Verification items for this drawing (mm, ordinates from the low corner). Give positions to 0.01 mm unless a question says otherwise; leave off trailing zeros. Loops run counter-clockwise (first coordinate to the right, second up) from the corner with the lowest first, then second, coordinate; pieces in that order, holes last. Notation, with made-up numbers: (46, 30.25) -> (50, 30.25) arc R11 cw to (50, 40.25) -> close; hole circle Ø11 at (77, 0.5). An arc over 180 degrees is marked (long way). Write item = value, one per line.
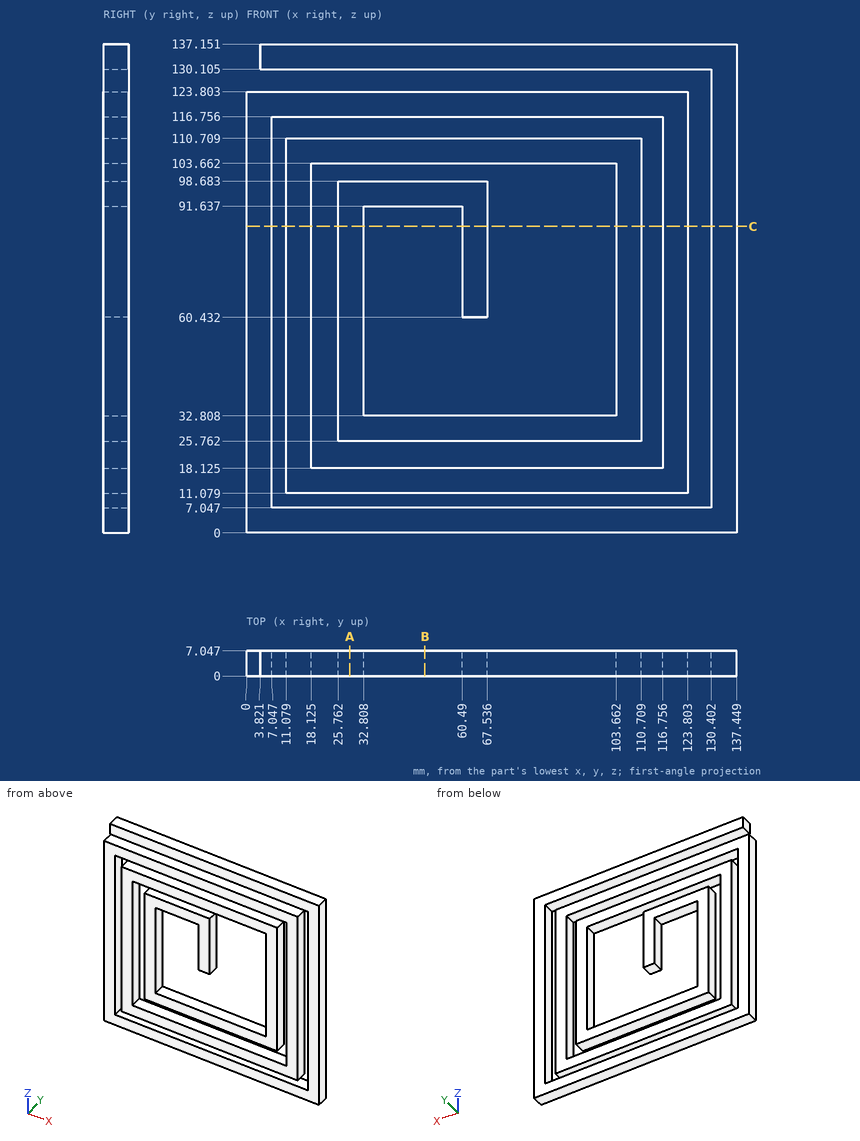
Item 1: Section check B-B, the plane x = 50. Record the cut outline in (y, z) (1 decimal).
Answer:
outline = (0, 0) -> (7, 0) -> (7, 7) -> (0, 7) -> close; (0, 11.1) -> (7, 11.1) -> (7, 18.1) -> (0, 18.1) -> close; (0, 25.8) -> (7, 25.8) -> (7, 32.8) -> (0, 32.8) -> close; (0, 91.6) -> (7, 91.6) -> (7, 98.7) -> (0, 98.7) -> close; (0, 103.7) -> (7, 103.7) -> (7, 110.7) -> (0, 110.7) -> close; (0, 116.8) -> (7, 116.8) -> (7, 123.8) -> (0, 123.8) -> close; (0, 130.1) -> (7, 130.1) -> (7, 137.2) -> (0, 137.2) -> close
Item 2: Section check A-A, the plane x = 29. Record the cut outline in (y, z) (1 decimal), plus the area to 3 significant figures.
Answer:
outline = (0, 0) -> (7, 0) -> (7, 7) -> (0, 7) -> close; (0, 11.1) -> (7, 11.1) -> (7, 18.1) -> (0, 18.1) -> close; (0, 25.8) -> (7, 25.8) -> (7, 98.7) -> (0, 98.7) -> close; (0, 103.7) -> (7, 103.7) -> (7, 110.7) -> (0, 110.7) -> close; (0, 116.8) -> (7, 116.8) -> (7, 123.8) -> (0, 123.8) -> close; (0, 130.1) -> (7, 130.1) -> (7, 137.2) -> (0, 137.2) -> close
area = 762 mm^2
Item 3: Section check C-C, the plane z = 86. Give the number of separate pieces and of enclosed holes in the cut face.
Answer:
separate_pieces = 7
enclosed_holes = 0
Item 4: Thickness scan on L1, parallel to Z at x = 71, y = 6 (1 decimal); L2, parallel to X at y = 6, z = 116; L3, parallel to Z at x = 18, y = 2 (1 decimal). Record the ranges inside material, lowest first. Write a range as [from, to].
Answer:
L1 = [0, 7], [11.1, 18.1], [25.8, 32.8], [103.7, 110.7], [116.8, 123.8], [130.1, 137.2]
L2 = [0, 7.05], [116.76, 123.8], [130.4, 137.45]
L3 = [0, 7], [11.1, 110.7], [116.8, 123.8], [130.1, 137.2]
